from build123d import *

# Parameters (mm, degrees)
F1_DEPTH = 9.525
F2_R     = 14.2748
F3_DEPTH = 25.4
F4_R     = 9.525


with BuildPart() as f1:
    # F0 (on Front) → F1 (new body)
    with BuildSketch(Plane.XZ):
        with BuildLine():
            Line((387.312791, 82.55), (-387.312791, 82.55))
            Line((-387.312791, 82.55), (-387.312791, 38.1))
            Line((-387.312791, 38.1), (-326.211106, -18.423178))
            ThreePointArc((-326.211106, -18.423178), (-316.509344, -24.556852), (-305.256305, -26.818544))
            Line((-305.256305, -26.818544), (-0.493514, -31.581044))
            ThreePointArc((-0.493514, -31.581044), (0, -31.5849), (0.493514, -31.581044))
            Line((0.493514, -31.581044), (305.256305, -26.818544))
            ThreePointArc((305.256305, -26.818544), (316.509344, -24.556852), (326.211106, -18.423178))
            Line((326.211106, -18.423178), (387.312791, 38.1))
            Line((387.312791, 38.1), (387.312791, 82.55))
        make_face()
    extrude(amount=F1_DEPTH)

    # F2 (on face) → F3 (cut)
    with BuildSketch(Plane.XZ.offset(9.525)):
        with Locations((-304.762791, 4.7625)):
            Circle(F2_R)
        Circle(F2_R)
        with Locations((304.762791, 4.7625)):
            Circle(F2_R)
        with BuildLine():
            Line((-309.525291, 76.2), (-380.962791, 76.2))
            Line((-380.962791, 76.2), (-380.962791, 40.876167))
            Line((-380.962791, 40.876167), (-324.021477, -11.798388))
            ThreePointArc((-324.021477, -11.798388), (-328.742633, 13.136695), (-309.525291, 29.712021))
            Line((-309.525291, 29.712021), (-309.525291, 76.2))
        make_face()
        with BuildLine():
            Line((-300.000291, 76.2), (-300.000291, 29.712021))
            ThreePointArc((-300.000291, 29.712021), (-281.230857, 14.323259), (-283.948798, -9.795581))
            Line((-283.948798, -9.795581), (-223.800291, 76.2))
            Line((-223.800291, 76.2), (-300.000291, 76.2))
        make_face()
    extrude(amount=-F3_DEPTH, mode=Mode.SUBTRACT)

    # F4
    f4_edges = [f1.edges().sort_by_distance(p)[0] for p in [
        (-300.000291, -4.7625, 29.712021),
        (-300.000291, -4.7625, 76.2),
        (-223.800291, -4.7625, 76.2),
        (-283.948798, -4.7625, -9.795581),
        (-309.525291, -4.7625, 29.712021),
        (-324.021477, -4.7625, -11.798388),
        (-380.962791, -4.7625, 40.876167),
        (-380.962791, -4.7625, 76.2),
        (-309.525291, -4.7625, 76.2),
    ]]
    fillet(f4_edges, radius=F4_R)


solid = f1.part
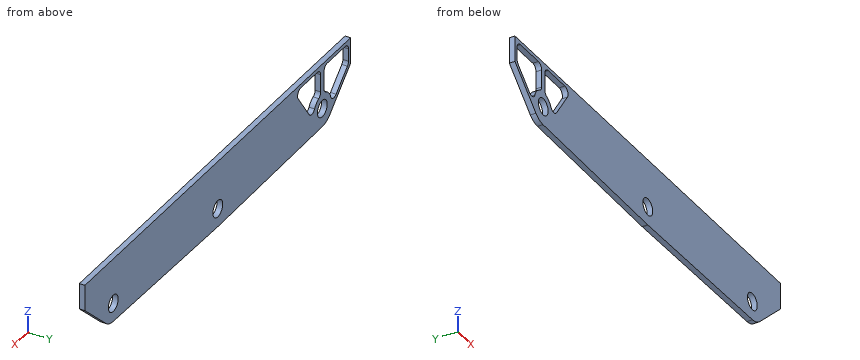
Geometry check sheet. Reference: the model listing, model coordinates, mm. Round coordinates to 2 decimals unless told otherwise and drop trailing zeros. Loops run counter-clockwise (first coordinate to the right, second up) from the corner with the lowest first, then second, coordinate; pieces in that order, holes last. Notation, with made-up numbers: (-29.5, 57.25) - (5.5, 57.25) arc R21 cw to (5.5, 79.25) - close; hole circle Ø5 at (71.25, 75.5). An arc over 180 degrees is marked (long way). One line per question, with ' | ' between items. Start each with the question number.
1. Cross-section at A-A on x = 143. Record the cut outline in (y, z) (3 decimals), then the cut area to 3 significant figures.
2. Depth check by flat-ended pin: pin 1 (5 mm diameter, centred on x = -341, y = -5.5, fed in from -Z); pin 2 (5 mm diameter, centred on x = -108.5, y = -1.5, fed in from -Z); pin 3 (3 mm diameter, centred on y = -5.5, z = 22, fed in from -X); pin 4 (1 mm diameter, centred on x = 230.5, z = 11.5, fed in from +Y). Enter the tip coordinate at first touch or a pass-through.
3. Scan lines: line 1 (X direction, y = -0.25, z = 44); line 2 (Z direction, x = -296, y = -0.5); line 3 (X direction, y = -4.75, z = 10.5). Record each from-to range of solid material in increasing order. Write a range as [from, to].
4. Cross-section at C-C on x = -122. Record the cut outline in (y, z) (3 decimals), then the cut area to 3 significant figures.
5. Cross-section at B-B on y = -5.5. State how many separate pieces and enclosed holes the cut face has, then the cut area to 3 significant figures.
Taken from the geometry:
1) outline: (-9.525, -29.354) - (0, -29.354) - (0, 82.55) - (-9.525, 82.55) - close | area: 1,070 mm²
2) pin 1: z = -7.06 | pin 2: z = -29.93 | pin 3: x = -371.53 | pin 4: y = 0
3) line 1: [-387.31, -380.91], [-309.53, -300], [-246.32, 387.31] | line 2: [-26.96, -6.51], [16.03, 28.87], [74.43, 82.55] | line 3: [-357.48, -348.13], [-329.64, -317.83], [-291.69, -9.67], [9.67, 291.69], [317.83, 357.48]
4) outline: (-9.525, -29.682) - (0, -29.682) - (0, 82.55) - (-9.525, 82.55) - close | area: 1,070 mm²
5) separate pieces: 1 | enclosed holes: 5 | area: 72,600 mm²
